CAD build for the part. Positions are in the model's coordinates, mm. Face numbers are marked on the shaded views. A direction names the side the tool comes from. Give positions to 0.01 mm unless a question says otherwise; leave off trailing zeros. Loops run counter-clockwise (first coordinate to the right, second up) from the corner with the lowest first, then second, coordinate; pieces in that order, holes last. Notation, with made-up numbers: M 71,12 L 85,12 A14 ccw 85,24 Z; hole C -37.5,49 d5. An arc over 180 degrees is marked long. Answer as CSV lines item,"result".
```python
from build123d import *

# Parameters (mm, degrees)
CROQUIS1_W              = 127
CROQUIS1_H              = 76.2
SALIENTE_EXTRUIR1_DEPTH = 25.4
CROQUIS2_W              = 101.6
CROQUIS2_H              = 62.484
CORTAR_EXTRUIR1_DEPTH   = 23.368
CORTAR_EXTRUIR2_REACH   = 137.003
CROQUIS3_W              = 46.736
CROQUIS3_H              = 15.688547189
CORTAR_EXTRUIR3_REACH   = 104.391
CORTAR_EXTRUIR4_REACH   = 137.003
CROQUIS5_W              = 5.1816
CROQUIS5_H              = 16.8021
CROQUIS5_W_2            = 16.03502
CROQUIS5_H_2            = 17.1196
CORTAR_EXTRUIR5_REACH   = 104.391
CROQUIS6_W              = 32.5628
CROQUIS6_H              = 19.05
CROQUIS7_R              = 2.4892
CORTAR_EXTRUIR6_DEPTH   = 79.288057838
CROQUIS8_W              = 5.207
CROQUIS8_H              = 5.207
SALIENTE_EXTRUIR2_DEPTH = 5.0038


with BuildPart() as part:
    # Croquis1 → Saliente-Extruir1 (new body)
    with BuildSketch(Plane(origin=(0, 0, 0), x_dir=(1, 0, 0), z_dir=(0, 1, 0))):
        Rectangle(CROQUIS1_W, CROQUIS1_H)
    extrude(amount=SALIENTE_EXTRUIR1_DEPTH)

    # Croquis2 → Cortar-Extruir1 (cut)
    with BuildSketch(Plane(origin=(0, 25.4, 0), x_dir=(1, 0, 0), z_dir=(0, 1, 0))):
        Rectangle(CROQUIS2_W, CROQUIS2_H)
    extrude(amount=-CORTAR_EXTRUIR1_DEPTH, mode=Mode.SUBTRACT)

    # Croquis3 → Cortar-Extruir2 (cut, up to next)
    with BuildSketch(Plane(origin=(63.5, 0, 0), x_dir=(0, 0, -1), z_dir=(1, 0, 0)), mode=Mode.PRIVATE) as cortar_extruir2_sk1:
        with Locations((0, 17.555726406)):
            Rectangle(CROQUIS3_W, CROQUIS3_H)
    cortar_extruir2_tool1 = extrude(cortar_extruir2_sk1.sketch, amount=-CORTAR_EXTRUIR2_REACH, mode=Mode.PRIVATE) & part.part
    add(cortar_extruir2_tool1.solids().sort_by_distance((63.5, 17.555726, 0))[0], mode=Mode.SUBTRACT)

    # Croquis4 → Cortar-Extruir3 (cut, up to next)
    with BuildSketch(Plane.XY.offset(38.1), mode=Mode.PRIVATE) as cortar_extruir3_sk1:
        Polygon((-37.592, 8.89), (17.78, 8.89), (17.78, 4.699), (37.592, 4.699), (37.592, 8.89), (37.592, 25.4), (-37.592, 25.4), align=None)
    cortar_extruir3_tool1 = extrude(cortar_extruir3_sk1.sketch, amount=-CORTAR_EXTRUIR3_REACH, mode=Mode.PRIVATE) & part.part
    add(cortar_extruir3_tool1.solids().sort_by_distance((1.735854, 16.496045, 38.1))[0], mode=Mode.SUBTRACT)

    # Croquis5 → Cortar-Extruir4 (cut, up to next)
    with BuildSketch(Plane.ZY.offset(63.5), mode=Mode.PRIVATE) as cortar_extruir4_sk1:
        with Locations((15.9512, 16.99895)):
            Rectangle(CROQUIS5_W, CROQUIS5_H)
    cortar_extruir4_tool1 = extrude(cortar_extruir4_sk1.sketch, amount=-CORTAR_EXTRUIR4_REACH, mode=Mode.PRIVATE) & part.part
    # Croquis5 → Cortar-Extruir4 (cut, up to next)
    with BuildSketch(Plane.ZY.offset(63.5), mode=Mode.PRIVATE) as cortar_extruir4_sk2:
        with Locations((-19.46529, 16.8402)):
            Rectangle(CROQUIS5_W_2, CROQUIS5_H_2)
    cortar_extruir4_tool2 = extrude(cortar_extruir4_sk2.sketch, amount=-CORTAR_EXTRUIR4_REACH, mode=Mode.PRIVATE) & part.part
    add(cortar_extruir4_tool1.solids().sort_by_distance((-63.5, 16.99895, 15.9512))[0], mode=Mode.SUBTRACT)
    add(cortar_extruir4_tool2.solids().sort_by_distance((-63.5, 16.8402, -19.46529))[0], mode=Mode.SUBTRACT)

    # Croquis6 → Cortar-Extruir5 (cut, up to next)
    with BuildSketch(Plane(origin=(0, 0, -38.1), x_dir=(-1, 0, 0), z_dir=(0, 0, -1)), mode=Mode.PRIVATE) as cortar_extruir5_sk1:
        with Locations((-21.8186, 11.8618)):
            Rectangle(CROQUIS6_W, CROQUIS6_H)
    cortar_extruir5_tool1 = extrude(cortar_extruir5_sk1.sketch, amount=-CORTAR_EXTRUIR5_REACH, mode=Mode.PRIVATE) & part.part
    add(cortar_extruir5_tool1.solids().sort_by_distance((21.8186, 11.8618, -38.1))[0], mode=Mode.SUBTRACT)

    # Croquis7 → Cortar-Extruir6 (cut, through all)
    with BuildSketch(Plane(origin=(0, 25.4, 0), x_dir=(1, 0, 0), z_dir=(0, 1, 0))):
        with BuildLine():
            ThreePointArc((-54.6608, 32.7914), (-57.15, 35.2806), (-59.6392, 32.7914))
            Line((-59.6392, 32.7914), (-54.6608, 32.7914))
        make_face()
        with BuildLine():
            Line((-54.6608, 32.7914), (-59.6392, 32.7914))
            ThreePointArc((-59.6392, 32.7914), (-57.15, 30.3022), (-54.6608, 32.7914))
        make_face()
        with Locations(Location((-57.15, -31.242, 0), (0, 0, 270))):
            Circle(CROQUIS7_R)
        with Locations(Location((57.15, 32.7914, 0), (0, 0, 270))):
            Circle(CROQUIS7_R)
        with Locations(Location((57.15, -31.242, 0), (0, 0, 270))):
            Circle(CROQUIS7_R)
    extrude(amount=-CORTAR_EXTRUIR6_DEPTH, mode=Mode.SUBTRACT)

    # Croquis8 → Saliente-Extruir2 (add)
    with BuildSketch(Plane(origin=(0, 2.032, 0), x_dir=(1, 0, 0), z_dir=(0, 1, 0))):
        with Locations((-48.1965, 28.6385)):
            Rectangle(CROQUIS8_W, CROQUIS8_H)
        with Locations((-48.1965, -28.6385)):
            Rectangle(CROQUIS8_W, CROQUIS8_H)
        with Locations((48.1965, -28.6385)):
            Rectangle(CROQUIS8_W, CROQUIS8_H)
        with Locations((48.1965, 28.6385)):
            Rectangle(CROQUIS8_W, CROQUIS8_H)
    extrude(amount=SALIENTE_EXTRUIR2_DEPTH)


solid = part.part
```
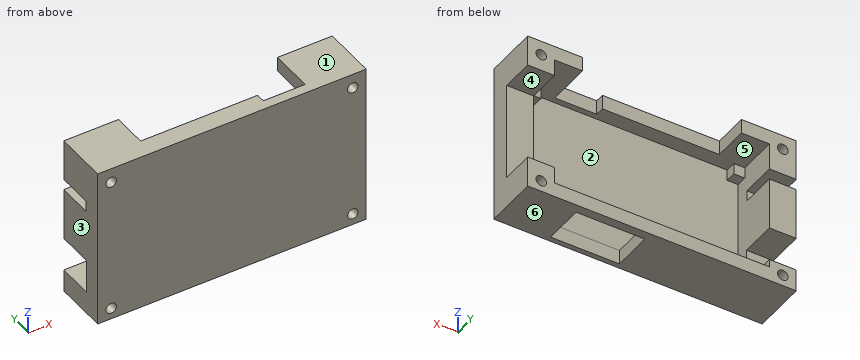
Q1. Mould opens along X. For the marked faces 1, 2 and 3 say: released by +X, released by -X, zero draft, split by the parting line, or undercut.
Solution:
face 1,"zero draft"
face 2,"undercut"
face 3,"released by -X"
Q2. Wall check: line 1 (X direction, y = 6.75, z = -26.5); line 2 (X direction, y = 2.75, z = 1.5); line 3 (X direction, y = 4.5, z = -34.5). Give the ranges that are in metal, low to high. Write a range as [from, to].
Solution:
line 1,"x = [-63.5, -45.59], [45.59, 63.5]"
line 2,"x = [-63.5, -50.8], [50.8, 63.5]"
line 3,"x = [-63.5, -58.96], [-55.34, 5.54], [38.1, 55.34], [58.96, 63.5]"
Q3. Pin check, flat tips, straight feed: P1, Ø10, axis at x = 17.5, y = 15.5, coming from the +Z side; P2, Ø1, axis at x = 16, z = -2.5, coming from the +Y side; P3, Ø2.5, axis at x = -49, z = 28.5, coming from the +Y side; P4, Ø4, axis at x = -54, z = -20, coming from the +Y side. Stop position of each tip, or through.
Solution:
P1,"passes through"
P2,"stops at y = 2.03"
P3,"stops at y = 7.04"
P4,"stops at y = 8.28"
Q4. Which spindle directions (+Z, -Z, +X, -X, +Y, -Y) get a long thin tool onto all of the face, cutting with end or side? Do the marked faces 4, 5 and 6. Say none if no direction does.
Solution:
face 4,"+X, +Y"
face 5,"+Y"
face 6,"-Z, +X, -X, +Y, -Y"
Q5. Cut at A-A (y = 11.5). Give the number of separate pieces and of enclosed holes in the cut face, and give its area (3 significant figures).
Solution:
separate pieces,"5"
enclosed holes,"4"
area,"1,650 mm²"
Q6. Cut at B-B (x = -57.15). Write the cut outline in (y, z), and give its area (3 significant figures).
Solution:
outline,"M 0,-38.1 L 25.4,-38.1 L 25.4,-35.28 L 0,-35.28 Z; M 0,-30.3 L 25.4,-30.3 L 25.4,-27.48 L 8.28,-27.48 L 8.28,-11.45 L 25.4,-11.45 L 25.4,13.36 L 8.6,13.36 L 8.6,18.54 L 25.4,18.54 L 25.4,28.75 L 0,28.75 Z; M 0,33.73 L 25.4,33.73 L 25.4,38.1 L 0,38.1 Z"
area,"1,320 mm²"
Q7. Cut at C-C (y = 23). Write the cut outline in (x, z).
Solution:
outline,"M -63.5,-38.1 L 63.5,-38.1 L 63.5,-23.37 L 50.8,-23.37 L 50.8,-31.24 L -50.8,-31.24 L -50.8,-27.48 L -63.5,-27.48 Z; M -63.5,-11.45 L -50.8,-11.45 L -50.8,13.36 L -63.5,13.36 Z; M -63.5,18.54 L -50.8,18.54 L -50.8,31.24 L -37.59,31.24 L -37.59,38.1 L -63.5,38.1 Z; M 37.59,31.24 L 50.8,31.24 L 50.8,23.37 L 63.5,23.37 L 63.5,38.1 L 37.59,38.1 Z; hole C -57.15,-32.79 d4.98; hole C -57.15,31.24 d4.98; hole C 57.15,-32.79 d4.98; hole C 57.15,31.24 d4.98"
Q8. Cut at D-D (x = 53). Write the cut outline in (y, z), and give its area (3 significant figures).
Solution:
outline,"M 0,-38.1 L 25.4,-38.1 L 25.4,-23.37 L 9.71,-23.37 L 9.71,23.37 L 25.4,23.37 L 25.4,38.1 L 0,38.1 Z"
area,"1,200 mm²"
